Answer from the drawing. Dimensions are ordinates in mm from the lowest x, y and z of the part. A direction names the side the tool comes from. Round coordinates to 2 decimals unless told otherwise and drop trailing zeros. Order: outer loops, then holes, each group sorted by start corner. A loop starts at its lowest first (then second) coordinate and runs counter-clockwise, first axis right, second up. Notation, with made-up numbers: (41.5, 72.5) -> (63.5, 72.5) arc R17 cw to (63.5, 104.5) -> close; hole circle Ø3 at (-13.5, 0.25). An arc over 180 degrees is marked (long way). Use a Markdown table: item, result. Add a question column.
Item 1: Find the intervals of material crossed by L1, parallel to Y at x = 8, z = 10; L2, parallel to Z at x = 10.5, y = 16; L3, parallel to Z at x = 22, y = 11, in increasing order. Write a range as [from, to].
Item 2: A cutting plane is placed at A-A, the plane y = 10. Determine the outline of the cut face in (x, z).
Item 3: Flat-ended cylindrical pins translate along their axes: P1, Ø1.1, axis at x = 25, y = 16.5, coming from the +Z side; P2, Ø1.5, axis at x = 4.5, y = 14, coming from the -Z side; P3, Ø1, axis at x = 31, y = 8, coming from the -Z side; P4, Ø9.5, axis at y = 10, z = 10, coming from the +X side. Find the tip coordinate at first contact, or state that the pin passes through.
Item 4: A tool of negligible diameter and unlimited length cuts with its end or side. For the marked faces 4 and 5, from which of +Z, -Z, +X, -X, +Y, -Y can it reach the whole face along a straight path? Write none if from no direction.
Item 5: A cutting plane is placed at C-C, the plane x = 21. Determine the outline of the cut face in (y, z), plus the area to 3 significant figures.
Item 6: A cutting plane is placed at B-B, the plane z = 10. Determine the outline of the cut face in (x, y).
Item 7: For a pull along Y with two mould halves and no side action, classify the marked faces 1, 2 and 3 as +Y half, -Y half, draft (parallel to the pull), parting line (faces both ways), or undercut.
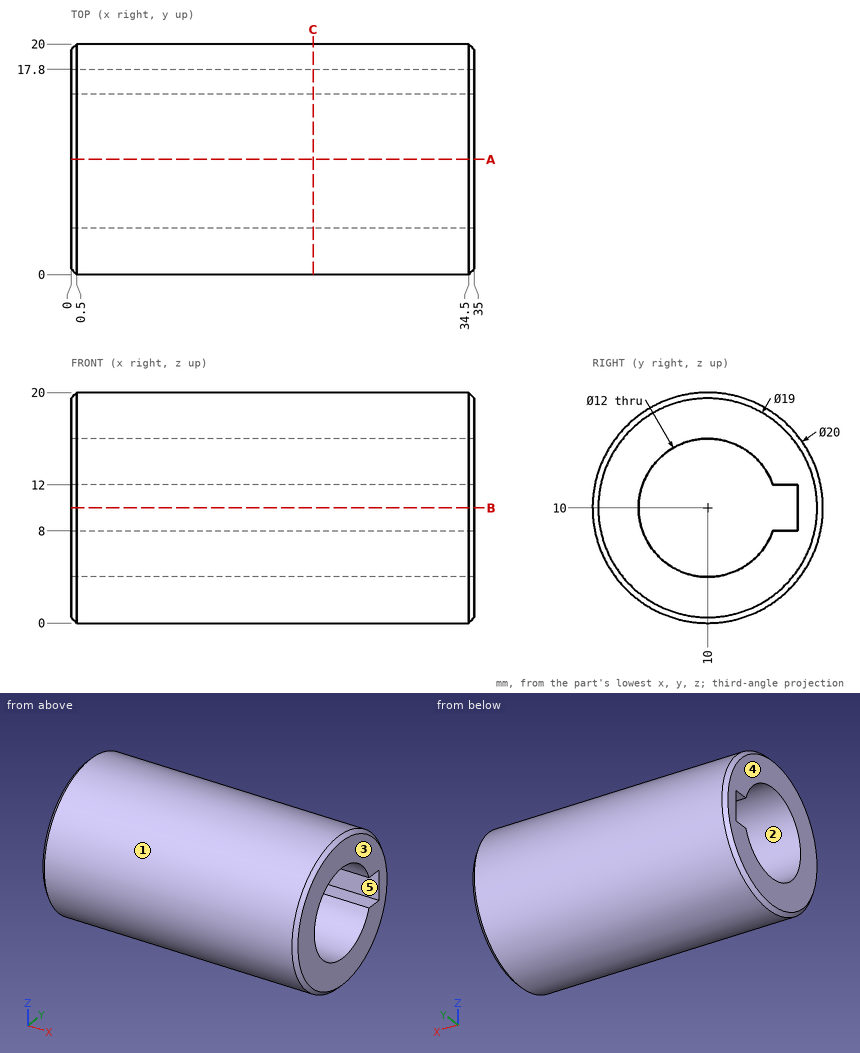
Reported:
| question | item | result |
|---|---|---|
| 1 | L1 | [0, 4], [17.8, 20] |
| 1 | L2 | [2, 8], [12, 18] |
| 1 | L3 | [0.05, 4.08], [15.92, 19.95] |
| 2 | outline | (0, 0.5) -> (0.5, 0) -> (34.5, 0) -> (35, 0.5) -> (35, 4) -> (0, 4) -> close; (0, 16) -> (35, 16) -> (35, 19.5) -> (34.5, 20) -> (0.5, 20) -> (0, 19.5) -> close |
| 3 | P1 | z = 18.04 |
| 3 | P2 | z = 0.54 |
| 3 | P3 | z = 0.11 |
| 3 | P4 | through |
| 4 | face 4 | +Z, -Z, -X, +Y, -Y |
| 4 | face 5 | +X, -X |
| 5 | outline | circle Ø20 at (10, 10); hole (15.66, 8) -> (17.8, 8) -> (17.8, 12) -> (15.66, 12) arc R6 ccw (long way) to start |
| 5 | area | 193 mm² |
| 6 | outline | (0, 0.5) -> (0.5, 0) -> (34.5, 0) -> (35, 0.5) -> (35, 4) -> (0, 4) -> close; (0, 17.8) -> (35, 17.8) -> (35, 19.5) -> (34.5, 20) -> (0.5, 20) -> (0, 19.5) -> close |
| 7 | face 1 | parting line |
| 7 | face 2 | undercut |
| 7 | face 3 | draft |
